Autodesk Fusion 360 part; units mm, degrees
sketch "Sketch5" plane through (0, 0, 0) normal (0, 0, 1) x (1, 0, 0)
  circle A0 centre (0, 0) radius 7.5
  line L0 (2.5, 2.0767) -> (2.5, -2.0767)
  arc A1 (2.5, 2.0767) -> (2.5, -2.0767) centre (0, 0) ccw
  dimension "d22" = 15
  dimension "d29" = 6.5
  dimension "d30" = 2.5
extrude "Extrude5" add sketch "Sketch5" along normal blind 10
sketch "Sketch6" plane through (0, 0, 10) normal (0, 0, 1) x (-1, 0, 0)
  circle A0 centre (0, 0) radius 7.5
  circle A1 centre (0, 0) radius 7.5
  arc A2 (-2.5, -2.0767) -> (-2.5, 2.0767) centre (0, 0) ccw
  line L0 (-2.5, -2.0767) -> (-2.5, 2.0767)
  line L1 (-2.7005, -3.2818) -> (-3.0882, 2.9198)
  arc A3 (-2.7005, -3.2818) -> (-3.0882, 2.9198) centre (0, 0) ccw
  dimension "d31" = 8.5
  dimension "d32" = 2.9
extrude "Extrude6" add sketch "Sketch6" along normal blind 10 contours A0 A1
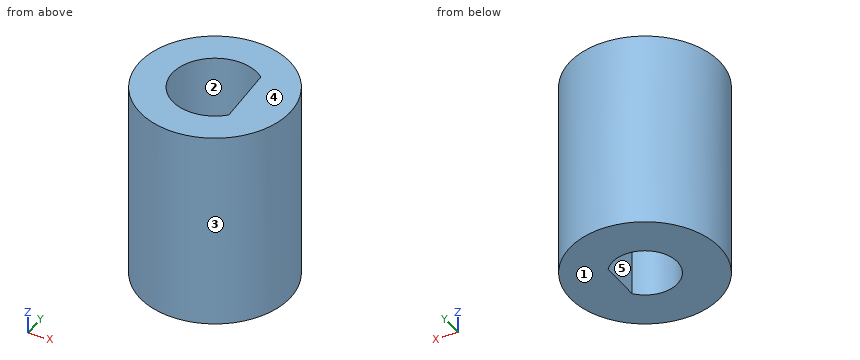
CAD build for the part. Positions are in the model's coordinates, mm. Face numbers are marked on the shaded views. A direction names the side the tool comes from. Round coordinates to 2 decimals unless told otherwise and drop trailing zeros. Loops run counter-clockwise (first coordinate to the right, second up) from the corner with the lowest first, then second, coordinate; pieces in that order, holes last. Notation, with made-up numbers: M 65,1 L 100,1 A13 ccw 100,16 Z; hole C 41.25,-30.5 d5. An arc over 180 degrees is marked long. Return JSON: item names as keys, results as strings. Group by question number.
(1) Tool access for the marked faces 1 and 2: list every direction of +Z, -Z, +X, -X, +Y, -Y with a clear straight run to the whole face (end or side of a thin tool).
(2) Wall check: probe 1 along Y at (x, z) = (0, 6.75); probe 2 along X at (y, z) = (0.25, 1.75); probe 3 along X at (y, z) = (2.75, 10.75). Give the ranges that are in metal, low to high. Write a range as [from, to].
(3) Mould opens along X. For the marked faces 3, 4 and 5 say: +X half, -X half, draft (parallel to the pull), parting line (faces both ways), or undercut.
(4) Saw through at C-C, the plane y = -4.75. List the corners of the cut face in (x, z).
(5) Saw through at B-B, the plane z = 17. List the corners of the cut face in (x, y), and give its area (3 significant figures).
(6) Drop flat-ended pins along their axis: P1, Ø6, axis at y = -3, z = 11, coming from the +X side; P2, Ø4, axis at x = 0, y = 0, coming from the -Z side; P3, Ø3.5, axis at x = -1.5, y = -1, coming from the +Z side; P4, Ø1.2, axis at y = -1, z = 4.5, coming from the -X side. Give the stop position or say it passes through.
Answer list:
{
 "1": {"face 1": "-Z, +X, -X, +Y, -Y", "face 2": "+Z"},
 "2": {"probe 1": "[-7.5, -3.25], [3.25, 7.5]", "probe 2": "[-7.5, -3.24], [2.5, 7.5]", "probe 3": "[-6.98, -3.24], [2.73, 6.98]"},
 "3": {"face 3": "parting line", "face 4": "draft", "face 5": "undercut"},
 "4": {"outline": "M -5.8,0 L 5.8,0 L 5.8,20 L -5.8,20 Z"},
 "5": {"outline": "C 0,0 d15; hole M 2.7,3.28 A4.25 ccw long 3.09,-2.92 Z", "area": "126 mm2"},
 "6": {"P1": "x = 7.5", "P2": "through", "P3": "z = 10", "P4": "x = -7.49"}
}
